Work out the finished part from the listing and answer in its coordinate system (mm). A direction names the side the tool comes from. Round coordinates to 2 decimals unless told otherwise and drop trailing zeros. Write each loop counter-clockwise with the first axis right and the second up, starting at its lowest first coordinate (ties: lowest second). Pieces come first, ordered by that corner, then holes. Notation, with made-up numbers: (-4, 39) -> (0, 39) arc R29 ccw to (0, 77) -> close; hole circle Ø7 at (5.25, 40). An arc over 180 degrees is marked (long way). One line per item, written item: value.
```python
from build123d import *

# Parameters (mm, degrees)
F1_DEPTH = 63.5
F2_DEPTH = 25.4
F0_W     = 25.4
F0_H     = 19.05
F3_DEPTH = 25.4
F4_DEPTH = 7.9375
F6_R     = 5.08


with BuildPart() as f1:
    # F0 (on Front) → F1 (new body, symmetric)
    with BuildSketch(Plane.XZ):
        Polygon((22.225, 9.525), (-41.275, 9.525), (-41.275, -9.525), (41.275, -9.525), (41.275, 9.525), align=None)
    extrude(amount=F1_DEPTH, both=True)

    # F0 (on Front) → F2 (join, symmetric)
    with BuildSketch(Plane.XZ):
        with BuildLine():
            Line((22.225, 27.0002), (22.225, 9.525))
            Line((22.225, 9.525), (41.275, 9.525))
            Line((41.275, 9.525), (41.275, 27.0002))
            ThreePointArc((41.275, 27.0002), (45.9246798487, 38.2255201513), (57.15, 42.8752))
            Line((57.15, 42.8752), (60.325, 42.8752))
            Line((60.325, 42.8752), (60.325, 61.9252))
            Line((60.325, 61.9252), (57.15, 61.9252))
            add(Edge.make_bspline(
                [(54.1922002544, 61.799726515), (55.2011160531, 61.8602288921), (56.1877673856, 61.9022138929), (57.15, 61.9252)],
                knots=[108.3505777535, 108.3505777535, 108.3505777535, 108.3505777535, 111.5045361635, 111.5045361635, 111.5045361635, 111.5045361635], degree=3))
            ThreePointArc((54.1922002544, 61.799726515), (31.4298057831, 50.627032933), (22.225, 27.0002))
        make_face()
    extrude(amount=F2_DEPTH, both=True)

    # F0 (on Front) → F3 (join, symmetric)
    with BuildSketch(Plane.XZ):
        with Locations((73.025, 52.4002)):
            Rectangle(F0_W, F0_H)
    extrude(amount=F3_DEPTH, both=True)

    # F0 (on Front) → F4 (join, symmetric)
    with BuildSketch(Plane.XZ):
        with BuildLine():
            add(Edge.make_bspline(
                [(-41.275, 9.525), (-41.4042765408, 35.7887962945), (19.5320698785, 59.7212376229), (54.1922002544, 61.799726515)],
                knots=[0, 0, 0, 0, 108.3505777535, 108.3505777535, 108.3505777535, 108.3505777535], degree=3))
            Line((-41.275, 9.525), (22.225, 9.525))
            Line((22.225, 9.525), (22.225, 27.0002))
            ThreePointArc((22.225, 27.0002), (31.4298057831, 50.627032933), (54.1922002544, 61.799726515))
        make_face()
    extrude(amount=F4_DEPTH, both=True)

    # F0 (on Front) → F5 (revolve)
    with BuildSketch(Plane.XZ):
        Polygon((85.725, 66.675), (85.725, 61.9252), (85.725, 42.8752), (85.725, 38.1), (111.125, 38.1), (111.125, 66.675), align=None)
    revolve(axis=Axis((85.725, 0, 52.3875), (0, 0, 1)))

    # F6
    f6_edges = [f1.edges().sort_by_distance(p)[0] for p in [
        (-41.275, -63.5, 0),
        (-41.275, 63.5, 0),
        (41.275, 63.5, 0),
        (41.275, -63.5, 0),
    ]]
    fillet(f6_edges, radius=F6_R)


solid = f1.part
```
(1) Find section B-B on y = 38.5. Give the vertices of the cut face in (x, z) (3 decimals).
Reported:
outline: (-41.275, -9.525) -> (41.275, -9.525) -> (41.275, 9.525) -> (-41.275, 9.525) -> close
(2) Find section A-A on z = -1.5. Give the vertices of the cut face in (x, y) (3 decimals).
Reported:
outline: (-41.275, -58.42) arc R5.08 ccw to (-36.195, -63.5) -> (36.195, -63.5) arc R5.08 ccw to (41.275, -58.42) -> (41.275, 58.42) arc R5.08 ccw to (36.195, 63.5) -> (-36.195, 63.5) arc R5.08 ccw to (-41.275, 58.42) -> close
(3) Find section C-C on x = 64. Give the vertices of the cut face in (y, z) (3 decimals), plus the area to 3 significant figures.
Reported:
outline: (-25.4, 42.875) -> (-13.16, 42.875) -> (-13.16, 38.1) -> (13.16, 38.1) -> (13.16, 42.875) -> (25.4, 42.875) -> (25.4, 61.925) -> (13.16, 61.925) -> (13.16, 66.675) -> (-13.16, 66.675) -> (-13.16, 61.925) -> (-25.4, 61.925) -> close
area: 1,220 mm2
(4) A tool of negligible diameter and unlimited length cuts with its end or side. For faces 5 (the face through (1, -36, 9.525)), 6 (the face through (46, -25.4, 42)), 7 (the face through (22.225, 17, 18)), 8 (the face through (46, 25.4, 42)), 9 (the face through (86, 0, 38.1)), from which of +Z, -Z, +X, -X, +Y, -Y can it reach the whole face along a straight path? Write none if from no direction.
Reported:
face 5: +Z, -X, -Y
face 6: +Z, +X, -X, -Y
face 7: +Z, -X, +Y
face 8: +Z, +X, -X, +Y
face 9: -Z, +X, +Y, -Y
(5) Consider probe 1 along X at (y, z) = (-50, -1) (3 decimals); probe 2 along Z at (x, y) = (99.5, 0) (3 decimals); probe 3 along Z at (x, y) = (16.5, 41) (3 decimals). Determine where each line is inside the solid, lowest interval first.
Reported:
probe 1: x = -41.275 to 41.275
probe 2: z = 38.1 to 66.675
probe 3: z = -9.525 to 9.525
(6) Flat-ended cylindrical pins translate along their axes: pin 1 Ø15.5 at (x, z) = (12.5, 36) entering from -Y; pin 2 Ø14.5 at (x, y) = (76.5, 0.5) entering from -Z; pin 3 Ø18.5 at (y, z) = (-12.5, 3) entering from +X (3 decimals); pin 4 Ø12 at (y, z) = (-1.5, 45.5) entering from +X (3 decimals). Find the tip coordinate at first contact, or state that the pin passes through.
Reported:
pin 1: stops at y = -7.94
pin 2: stops at z = 38.1
pin 3: stops at x = 41.275
pin 4: stops at x = 111.125
(7) For a pull along X with two mould halves and no side action, classify faces 1 (the face through (60, 2, 42.875)), 2 (the face through (60, 2, 61.925)), 3 (the face through (41.275, -1, 4)), 4 (the face through (45.8, -0.4, 38.1)) as pulls with the +X half, pulls with the -X half, needs draft (parallel to the pull), parting line crosses it, or undercut.
Reported:
face 1: undercut
face 2: needs draft
face 3: pulls with the +X half
face 4: undercut
